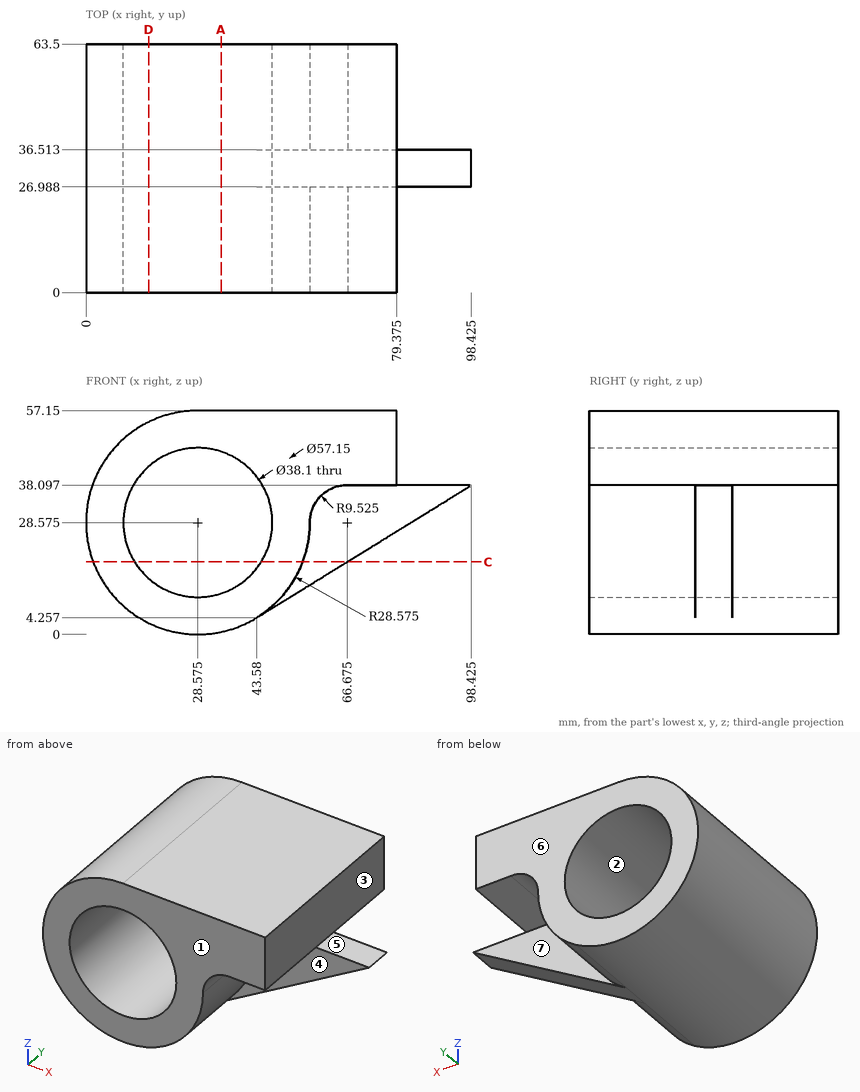
Check sheet for the drawn part. Datum: minimum x, y, z corner. Units: mm. A direction names the side the tool comes from. Coordinates: 2 decimals unless noted, no trailing zeros. Write each loop counter-clockwise with the first axis right and the second up, starting at its lowest first coordinate (ties: lowest second). Pieces come first, ordered by that corner, then holes. Notation, with made-up numbers: (-39, 36) - (12, 36) arc R13 ccw to (12, 41) - close; hole circle Ø7 at (74, -25.75). An arc over 180 degrees is marked (long way). Answer as a JSON object with one key per item and string values.
(1) Cross-section at D-D on x = 16. Record the cut outline in (y, z) (1 decimal).
Report:
{"outline": "(0, 2.9) - (63.5, 2.9) - (63.5, 14.3) - (0, 14.3) - close; (0, 42.9) - (63.5, 42.9) - (63.5, 54.2) - (0, 54.2) - close"}
(2) Tool access check on the marked faces 4, 5, 6 and 7. Record the directions out of +Z, -Z, +X, -X, +Y, -Y that give a thin tool (end or side, any length) a straight path to the whole face; none if there is none.
Report:
{"face 4": "-Z, +X, -Y", "face 5": "+Z, +X, +Y, -Y", "face 6": "+Z, -Z, +X, -X, +Y", "face 7": "-Z, +X, +Y"}
(3) Cross-section at C-C on z = 18.5. Record the cut outline in (x, y) (1 decimal).
Report:
{"outline": "(1.8, 0) - (12.4, 0) - (12.4, 63.5) - (1.8, 63.5) - close; (44.7, 0) - (55.3, 0) - (55.3, 27) - (66.7, 27) - (66.7, 36.5) - (55.3, 36.5) - (55.3, 63.5) - (44.7, 63.5) - close"}
(4) Gauge pin test, flat ends, axial feed: pin 1 Ø10 at (x, y) = (70.5, 7.5) entering from -Z; pin 2 Ø10 at (x, z) = (66, 17) entering from -Y; pin 3 Ø2 at (x, y) = (35.5, 28.5) entering from -Z; pin 4 Ø6 at (x, y) = (88, 40.5) entering from -Z. Record the tip position at first contact, or that the pin passes through.
Report:
{"pin 1": "z = 38.03", "pin 2": "y = 26.99", "pin 3": "z = 0.62", "pin 4": "through"}
(5) Thickness scan on line 1 along X through (y, z) = (56, 29); line 2 along X through (y, z) = (16, 41) (1 decimal); line 3 along Z through (x, y) = (31, 24). Record the ranges inside material, lowest first.
Report:
{"line 1": "0 to 9.53, 47.62 to 57.16", "line 2": "2.8 to 14.1, 43 to 79.4", "line 3": "0.1 to 9.68, 47.47 to 57.15"}
(6) Mould release check, pull along X, two halves, no side actions. Record for the marked faces 1, 2 and 3: pulls with the +X half, pulls with the -X half, needs draft (parallel to the pull), parting line crosses it, or undercut.
Report:
{"face 1": "needs draft", "face 2": "undercut", "face 3": "pulls with the +X half"}
(7) Cross-section at A-A on x = 34.5. Record the cut outline in (y, z), plus the area to 3 significant figures.
Report:
{"outline": "(0, 0.62) - (63.5, 0.62) - (63.5, 10.47) - (0, 10.47) - close; (0, 46.68) - (63.5, 46.68) - (63.5, 57.15) - (0, 57.15) - close", "area": "1,290 mm^2"}
